```python
from build123d import *

# Parameters (mm, degrees)
SKETCH2_R               = 18
SKETCH2_W               = 7.5
SKETCH2_H               = 7.5
BOSS_EXTRUDE1_DEPTH     = 1.3
BOSS_EXTRUDE10_START    = 1.3
SKETCH18_W              = 7.7
SKETCH18_H              = 7.7
BOSS_EXTRUDE10_DEPTH    = 1.3
BOSS_EXTRUDE2_START     = -1.3
SKETCH3_R               = 35
SKETCH3_R_2             = 18
BOSS_EXTRUDE2_DEPTH     = 1.3
CUT_EXTRUDE1_DEPTH      = 50.514543318
CUT_EXTRUDE1_DEPTH_BACK = 50.514543318
SKETCH7_R               = 59.131365533
FILLET1_R               = 6
SKETCH4_R               = 3.2
CUT_EXTRUDE2_DEPTH      = 10


with BuildPart() as part:
    # Sketch2 → Boss-Extrude1 (new body)
    with BuildSketch(Plane.XY.offset(10)):
        Circle(SKETCH2_R)
        with BuildLine():
            Line((-8.15, -8.35), (-8.15, -14.91903147))
            ThreePointArc((-8.15, -14.91903147), (-11.939670478, -12.101415986), (-14.808021475, -8.35))
            Line((-14.808021475, -8.35), (-8.15, -8.35))
        make_face(mode=Mode.SUBTRACT)
        with BuildLine():
            Line((-8.15, -7.85), (-15.079041747, -7.85))
            ThreePointArc((-15.079041747, -7.85), (-16.470304718, -4.210589327), (-16.996396677, -0.35))
            Line((-16.996396677, -0.35), (-8.15, -0.35))
            Line((-8.15, -0.35), (-8.15, -7.85))
        make_face(mode=Mode.SUBTRACT)
        with BuildLine():
            Line((-8.15, 0.15), (-16.999338222, 0.15))
            ThreePointArc((-16.999338222, 0.15), (-16.521617742, 4.00451585), (-15.181485435, 7.65))
            Line((-15.181485435, 7.65), (-8.15, 7.65))
            Line((-8.15, 7.65), (-8.15, 0.15))
        make_face(mode=Mode.SUBTRACT)
        with BuildLine():
            Line((-8.15, 8.15), (-14.91903147, 8.15))
            ThreePointArc((-14.91903147, 8.15), (-12.02081528, 12.02081528), (-8.15, 14.91903147))
            Line((-8.15, 14.91903147), (-8.15, 8.15))
        make_face(mode=Mode.SUBTRACT)
        with BuildLine():
            Line((-7.65, 8.15), (-7.65, 15.181485435))
            ThreePointArc((-7.65, 15.181485435), (-4.00451585, 16.521617742), (-0.15, 16.999338222))
            Line((-0.15, 16.999338222), (-0.15, 8.15))
            Line((-0.15, 8.15), (-7.65, 8.15))
        make_face(mode=Mode.SUBTRACT)
        with BuildLine():
            Line((0.35, 8.15), (0.35, 16.996396677))
            ThreePointArc((0.35, 16.996396677), (4.210589327, 16.470304718), (7.85, 15.079041747))
            Line((7.85, 15.079041747), (7.85, 8.15))
            Line((7.85, 8.15), (0.35, 8.15))
        make_face(mode=Mode.SUBTRACT)
        with BuildLine():
            Line((8.35, 8.15), (8.35, 14.808021475))
            ThreePointArc((8.35, 14.808021475), (12.101415986, 11.939670478), (14.91903147, 8.15))
            Line((14.91903147, 8.15), (8.35, 8.15))
        make_face(mode=Mode.SUBTRACT)
        with BuildLine():
            Line((8.35, 7.65), (15.181485435, 7.65))
            ThreePointArc((15.181485435, 7.65), (16.521617742, 4.00451585), (16.999338222, 0.15))
            Line((16.999338222, 0.15), (8.35, 0.15))
            Line((8.35, 0.15), (8.35, 7.65))
        make_face(mode=Mode.SUBTRACT)
        with BuildLine():
            Line((8.35, -0.35), (16.996396677, -0.35))
            ThreePointArc((16.996396677, -0.35), (16.470304718, -4.210589327), (15.079041747, -7.85))
            Line((15.079041747, -7.85), (8.35, -7.85))
            Line((8.35, -7.85), (8.35, -0.35))
        make_face(mode=Mode.SUBTRACT)
        with BuildLine():
            Line((8.35, -8.35), (14.808021475, -8.35))
            ThreePointArc((14.808021475, -8.35), (12.02081528, -12.02081528), (8.35, -14.808021475))
            Line((8.35, -14.808021475), (8.35, -8.35))
        make_face(mode=Mode.SUBTRACT)
        with BuildLine():
            Line((7.85, -8.35), (7.85, -15.079041747))
            ThreePointArc((7.85, -15.079041747), (4.210589327, -16.470304718), (0.35, -16.996396677))
            Line((0.35, -16.996396677), (0.35, -8.35))
            Line((0.35, -8.35), (7.85, -8.35))
        make_face(mode=Mode.SUBTRACT)
        with BuildLine():
            Line((-0.15, -8.35), (-0.15, -16.999338222))
            ThreePointArc((-0.15, -16.999338222), (-4.00451585, -16.521617742), (-7.65, -15.181485435))
            Line((-7.65, -15.181485435), (-7.65, -8.35))
            Line((-7.65, -8.35), (-0.15, -8.35))
        make_face(mode=Mode.SUBTRACT)
        with Locations((-3.9, -4.1)):
            Rectangle(SKETCH2_W, SKETCH2_H, mode=Mode.SUBTRACT)
        with Locations((4.1, -4.1)):
            Rectangle(SKETCH2_W, SKETCH2_H, mode=Mode.SUBTRACT)
        with Locations((-3.9, 3.9)):
            Rectangle(SKETCH2_W, SKETCH2_H, mode=Mode.SUBTRACT)
        with Locations((4.1, 3.9)):
            Rectangle(SKETCH2_W, SKETCH2_H, mode=Mode.SUBTRACT)
    extrude(amount=-BOSS_EXTRUDE1_DEPTH)

    # Sketch18 → Boss-Extrude10 (add)
    with BuildSketch(Plane.XY.offset(8.7).offset(BOSS_EXTRUDE10_START)):
        with BuildLine():
            ThreePointArc((7.85, 15.079041747), (4.11362184, 16.494790552), (0.15, 16.999338222))
            Line((0.15, 16.999338222), (0.15, 8.15))
            Line((0.15, 8.15), (7.85, 8.15))
            Line((7.85, 8.15), (7.85, 15.079041747))
        make_face()
        with BuildLine():
            Line((8.15, 0.15), (16.999338222, 0.15))
            ThreePointArc((16.999338222, 0.15), (16.494790552, 4.11362184), (15.079041747, 7.85))
            Line((15.079041747, 7.85), (8.15, 7.85))
            Line((8.15, 7.85), (8.15, 0.15))
        make_face()
        with Locations((-4, 4)):
            Rectangle(SKETCH18_W, SKETCH18_H)
        with Locations((4, -4)):
            Rectangle(SKETCH18_W, SKETCH18_H)
        with BuildLine():
            Line((8.15, -8.15), (8.15, -14.91903147))
            ThreePointArc((8.15, -14.91903147), (12.02081528, -12.02081528), (14.91903147, -8.15))
            Line((14.91903147, -8.15), (8.15, -8.15))
        make_face()
        with BuildLine():
            Line((-7.85, -8.15), (-7.85, -15.079041747))
            ThreePointArc((-7.85, -15.079041747), (-4.11362184, -16.494790552), (-0.15, -16.999338222))
            Line((-0.15, -16.999338222), (-0.15, -8.15))
            Line((-0.15, -8.15), (-7.85, -8.15))
        make_face()
        with BuildLine():
            ThreePointArc((-16.999338222, -0.15), (-16.494790552, -4.11362184), (-15.079041747, -7.85))
            Line((-15.079041747, -7.85), (-8.15, -7.85))
            Line((-8.15, -7.85), (-8.15, -0.15))
            Line((-8.15, -0.15), (-16.999338222, -0.15))
        make_face()
        with BuildLine():
            ThreePointArc((-8.15, 14.91903147), (-12.02081528, 12.02081528), (-14.91903147, 8.15))
            Line((-14.91903147, 8.15), (-8.15, 8.15))
            Line((-8.15, 8.15), (-8.15, 14.91903147))
        make_face()
    extrude(amount=-BOSS_EXTRUDE10_DEPTH)

    # Sketch3 → Boss-Extrude2 (add)
    with BuildSketch(Plane(origin=(0, 0, 8.7), x_dir=(-1, 0, 0), z_dir=(0, 0, -1)).offset(BOSS_EXTRUDE2_START)):
        Circle(SKETCH3_R)
        Circle(SKETCH3_R_2, mode=Mode.SUBTRACT)
    extrude(amount=BOSS_EXTRUDE2_DEPTH)

    # Sketch7 → Cut-Extrude1 (cut, two sides: drawn at the far end of the back side and taken through both)
    with BuildSketch(Plane(origin=(0, 0, 8.7), x_dir=(-1, 0, 0), z_dir=(0, 0, -1)).offset(-CUT_EXTRUDE1_DEPTH_BACK)):
        Circle(SKETCH7_R)
        Polygon((0, 42), (-36.373066959, -21), (36.373066959, -21), align=None, mode=Mode.SUBTRACT)
    extrude(amount=CUT_EXTRUDE1_DEPTH + CUT_EXTRUDE1_DEPTH_BACK, mode=Mode.SUBTRACT)

    # Fillet1
    fillet1_edges = [part.edges().sort_by_distance(p)[0] for p in [
        (4.186533479, 34.748711306, 9.35),
        (32.186533479, -13.748711306, 9.35),
        (28, -21, 9.35),
        (-28, -21, 9.35),
        (-32.186533479, -13.748711306, 9.35),
        (-4.186533479, 34.748711306, 9.35),
    ]]
    fillet(fillet1_edges, radius=FILLET1_R)

    # Sketch4 → Cut-Extrude2 (cut)
    with BuildSketch(Plane(origin=(0, 0, 8.7), x_dir=(-1, 0, 0), z_dir=(0, 0, -1))):
        with Locations((0, 29)):
            Circle(SKETCH4_R)
        with Locations((25.11473671, -14.5)):
            Circle(SKETCH4_R)
        with Locations((-25.11473671, -14.5)):
            Circle(SKETCH4_R)
    extrude(amount=-CUT_EXTRUDE2_DEPTH, mode=Mode.SUBTRACT)


solid = part.part
```
The model under review builds one solid part; all positions refer to its coordinate system, in mm. A direction names the side the tool comes from. Coordinates: 2 decimals unless noted, no trailing zeros. Write each loop counter-clockwise with the first axis right and the second up, starting at its lowest first coordinate (ties: lowest second). Pieces come first, ordered by that corner, then holes.
1) We need section B-B on x = 14. State the section outline as (y, z) points.
2) Clearance check with a flat-ended pin moving along its axis: pin 1 Ø7.5 at (x, y) = (25.11, -14.5) entering from +Z. State where the tip first meets the part, or that it passes through.
3) We need section C-C on y = 11.5. State the section outline as (x, z) points, then the cut area to 3 significant figures.
4) We need section A-A on y = 29. State the section outline as (x, z) points.
5) To check wall thickness, follow probe 1 along Y at (x, z) = (3.5, 9.8); probe 2 along X at (y, z) = (-8.5, 9.4); probe 3 along Y at (x, z) = (-5.5, 9.2). State the ranges of each line that lie inside material, in increasing order.
6) The part is to be moulded in two halves that separate along Y. For faces 3 (the face through (-7.65, -4, 9)), 4 (the face through (-27.805, -20.205, 9.359)), 5 (the face through (0, 35, 9)), say which applies: pulls with the +Y half, pulls with the -Y half, needs draft (parallel to the pull), parting line crosses it, or undercut.
7) Machinability: for faces 1 (the face through (-18.36, 10.2, 9.36)), 2 (the face through (4, 0.15, 9)), which of the approach directions +Z, -Z, +X, -X, +Y, -Y give a long, thin tool a straight path to every point of the face, cutting with its end or side? Answer none if there is none.
8) We need section D-D on z = 9.2. Count the separate pieces of the cut face and the enclosed holes in it, then the cut area to 3 significant figures.
Answer list:
1. outline: (-21, 8.7) - (-7.85, 8.7) - (-7.85, 10) - (-21, 10) - close; (-0.35, 8.7) - (8.15, 8.7) - (8.15, 10) - (-0.35, 10) - close; (9.64, 8.7) - (17.75, 8.7) - (17.75, 10) - (9.64, 10) - close
2. pin 1: stops at z = 10
3. outline: (-17.61, 8.7) - (-7.65, 8.7) - (-7.65, 10) - (-17.61, 10) - close; (-0.15, 8.7) - (8.35, 8.7) - (8.35, 10) - (-0.15, 10) - close; (12.52, 8.7) - (17.61, 8.7) - (17.61, 10) - (12.52, 10) - close
3. area: 30.6 mm2
4. outline: (-7.51, 8.7) - (-3.2, 8.7) - (-3.2, 10) - (-7.51, 10) - close; (3.2, 8.7) - (7.51, 8.7) - (7.51, 10) - (3.2, 10) - close
5. probe 1: y = -21 to -16.64, -8.35 to 0.15, 7.65 to 34.24
5. probe 2: x = -29.16 to -14.72, -8.15 to 0.35, 7.85 to 29.16
5. probe 3: y = -21 to -7.85, -0.35 to 8.15, 16.09 to 32.43
6. face 3: undercut
6. face 4: pulls with the -Y half
6. face 5: pulls with the +Y half
7. face 1: +Z, -Z, -X, +Y
7. face 2: +Z, -Z
8. separate pieces: 1
8. enclosed holes: 11
8. area: 1,690 mm2
